Geometry check sheet. Reference: the model listing, model coordinates, mm. Face numbers are marked on the shaded views. A direction names the side the tool comes from. Coordinates: 2 decimals unless noted, no trailing zeros. Loops run counter-clockwise (first coordinate to the right, second up) from the corner with the lowest first, then second, coordinate; pieces in that order, holes last. Notation, with made-up numbers: (68, 33.25) - (87, 33.25) arc R19 cw to (87, 56.25) - close; hole circle Ø9 at (25, -24.5). An arc over 180 degrees is marked (long way). Write each question's results on one line, items separated by ' | '. Start each with the question number.
(1) Sectioned sample at B-B (x = -40). Enter the section's corners in (y, z), plus the area to 3 significant figures.
(2) Access from +Z, -Z, +X, -X, +Y, -Y to the whole of each face (thin tool, end or side, straight path). Record for the marked faces 1, 2 and 3.
(3) Mould release check, pull along X, two halves, no side actions. Record for the marked faces 4, 5 and 6: pulls with the +X half, pulls with the -X half, needs draft (parallel to the pull), parting line crosses it, or undercut.
(4) Go/stop test with flat-tipped pins: pin 1 Ø1 at (x, z) = (-74, 23) entering from -Y; pin 2 Ø13.5 at (y, z) = (-4, 31.5) entering from -X; pin 3 Ø10 at (x, z) = (-61.5, 13.5) entering from -Y. Record where each tip stops, or that it passes through.
(5) Sectioned sample at A-A (y = -24). Enter the section's corners in (x, z), plus the area to 3 significant figures.
(6) Material ranges on probe 1 along Y at (x, z) = (-90, 5.5); probe 2 along X at (y, z) = (-3, 16); probe 3 along X at (y, z) = (-11, 6), recorded low to high.
(7) Sectioned sample at C-C (z = 33). Enter the section's corners in (x, y), plus the area to 3 significant figures.
from build123d import *

# Parameters (mm, degrees)
F1_DEPTH = 40
F2_DEPTH = 10
F3_R     = 3
F4_SIZE  = 0.4
F5_SIZE  = 1


with BuildPart() as f1:
    # F0 (on Top) → F1 (new body)
    with BuildSketch(Plane.XY):
        with BuildLine():
            Line((-32.408465, 29.689309), (-97.408465, 29.689309))
            ThreePointArc((-97.408465, 29.689309), (-100.943999, 28.224843), (-102.408465, 24.689309))
            Line((-102.408465, 24.689309), (-102.408465, -35.310691))
            ThreePointArc((-102.408465, -35.310691), (-100.943999, -38.846224), (-97.408465, -40.310691))
            Line((-97.408465, -40.310691), (-32.408465, -40.310691))
            ThreePointArc((-32.408465, -40.310691), (-28.872931, -38.846224), (-27.408465, -35.310691))
            Line((-27.408465, -35.310691), (-27.408465, 24.689309))
            ThreePointArc((-27.408465, 24.689309), (-28.872931, 28.224843), (-32.408465, 29.689309))
        make_face()
        with BuildLine():
            Line((-101.408465, -34.310691), (-101.408465, 23.689309))
            ThreePointArc((-101.408465, 23.689309), (-99.943999, 27.224843), (-96.408465, 28.689309))
            Line((-96.408465, 28.689309), (-33.408465, 28.689309))
            ThreePointArc((-33.408465, 28.689309), (-29.872931, 27.224843), (-28.408465, 23.689309))
            Line((-28.408465, 23.689309), (-28.408465, -34.310691))
            ThreePointArc((-28.408465, -34.310691), (-29.872931, -37.846224), (-33.408465, -39.310691))
            Line((-33.408465, -39.310691), (-96.408465, -39.310691))
            ThreePointArc((-96.408465, -39.310691), (-99.943999, -37.846224), (-101.408465, -34.310691))
        make_face(mode=Mode.SUBTRACT)
    extrude(amount=F1_DEPTH)

    # F0 (on Top) → F2 (join)
    with BuildSketch(Plane.XY):
        with BuildLine():
            Line((-24.408465, 37.689309), (-105.408465, 37.689309))
            ThreePointArc((-105.408465, 37.689309), (-108.943999, 36.224843), (-110.408465, 32.689309))
            Line((-110.408465, 32.689309), (-110.408465, -43.310691))
            ThreePointArc((-110.408465, -43.310691), (-108.943999, -46.846224), (-105.408465, -48.310691))
            Line((-105.408465, -48.310691), (-24.408465, -48.310691))
            ThreePointArc((-24.408465, -48.310691), (-20.872931, -46.846224), (-19.408465, -43.310691))
            Line((-19.408465, -43.310691), (-19.408465, 32.689309))
            ThreePointArc((-19.408465, 32.689309), (-20.872931, 36.224843), (-24.408465, 37.689309))
        make_face()
        with BuildLine():
            Line((-105.408465, -38.310691), (-105.408465, 27.689309))
            ThreePointArc((-105.408465, 27.689309), (-103.943999, 31.224843), (-100.408465, 32.689309))
            Line((-100.408465, 32.689309), (-29.408465, 32.689309))
            ThreePointArc((-29.408465, 32.689309), (-25.872931, 31.224843), (-24.408465, 27.689309))
            Line((-24.408465, 27.689309), (-24.408465, -38.310691))
            ThreePointArc((-24.408465, -38.310691), (-25.872931, -41.846224), (-29.408465, -43.310691))
            Line((-29.408465, -43.310691), (-100.408465, -43.310691))
            ThreePointArc((-100.408465, -43.310691), (-103.943999, -41.846224), (-105.408465, -38.310691))
        make_face(mode=Mode.SUBTRACT)
        with BuildLine():
            ThreePointArc((-100.408465, 32.689309), (-103.943999, 31.224843), (-105.408465, 27.689309))
            Line((-105.408465, 27.689309), (-105.408465, -38.310691))
            ThreePointArc((-105.408465, -38.310691), (-103.943999, -41.846224), (-100.408465, -43.310691))
            Line((-100.408465, -43.310691), (-29.408465, -43.310691))
            ThreePointArc((-29.408465, -43.310691), (-25.872931, -41.846224), (-24.408465, -38.310691))
            Line((-24.408465, -38.310691), (-24.408465, 27.689309))
            ThreePointArc((-24.408465, 27.689309), (-25.872931, 31.224843), (-29.408465, 32.689309))
            Line((-29.408465, 32.689309), (-100.408465, 32.689309))
        make_face()
        with BuildLine():
            ThreePointArc((-102.408465, 24.689309), (-100.943999, 28.224843), (-97.408465, 29.689309))
            Line((-97.408465, 29.689309), (-32.408465, 29.689309))
            ThreePointArc((-32.408465, 29.689309), (-28.872931, 28.224843), (-27.408465, 24.689309))
            Line((-27.408465, 24.689309), (-27.408465, -35.310691))
            ThreePointArc((-27.408465, -35.310691), (-28.872931, -38.846224), (-32.408465, -40.310691))
            Line((-32.408465, -40.310691), (-97.408465, -40.310691))
            ThreePointArc((-97.408465, -40.310691), (-100.943999, -38.846224), (-102.408465, -35.310691))
            Line((-102.408465, -35.310691), (-102.408465, 24.689309))
        make_face(mode=Mode.SUBTRACT)
    extrude(amount=F2_DEPTH)

    # F3
    f3_edges = [f1.edges().sort_by_distance(p)[0] for p in [
        (-64.908465, -40.310691, 10),
        (-64.908465, -48.310691, 10),
        (-64.908465, -48.310691, 0),
    ]]
    fillet(f3_edges, radius=F3_R)

    # F4
    f4_edges = [f1.edges().sort_by_distance(p)[0] for p in [
        (-64.908465, -40.310691, 40),
        (-64.908465, -39.310691, 40),
    ]]
    chamfer(f4_edges, length=F4_SIZE)

    # F5
    f5_edges = [f1.edges().sort_by_distance(p)[0] for p in [
        (-101.408465, -5.310691, 0),
    ]]
    chamfer(f5_edges, length=F5_SIZE)


solid = f1.part
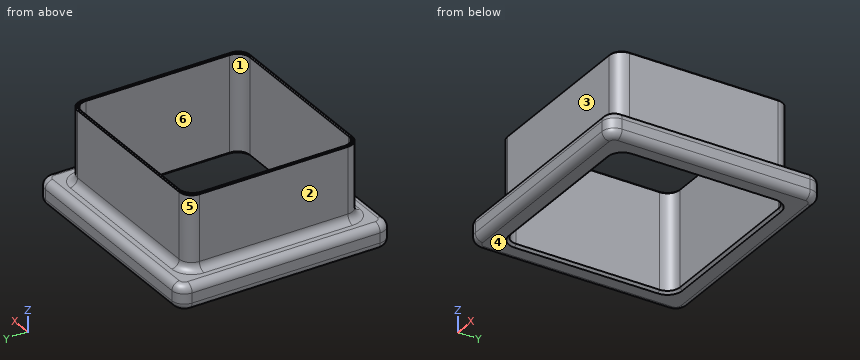
Outcome:
1) outline: (-48.31, 3) arc R3 ccw to (-45.31, 0) - (-40.31, 0) - (-39.31, 1) - (-39.31, 39.6) - (-39.71, 40) - (-39.91, 40) - (-40.31, 39.6) - (-40.31, 13) arc R3 cw to (-43.31, 10) - (-45.31, 10) arc R3 ccw to (-48.31, 7) - close; (28.69, 1) - (29.69, 0) - (34.69, 0) arc R3 ccw to (37.69, 3) - (37.69, 7) arc R3 ccw to (34.69, 10) - (32.69, 10) arc R3 cw to (29.69, 13) - (29.69, 39.6) - (29.29, 40) - (29.09, 40) - (28.69, 39.6) - close | area: 235 mm2
2) face 1: +Z, -Z | face 2: +Z, -X, +Y, -Y | face 3: +Z, +X, -X, -Y
3) face 4: needs draft | face 5: pulls with the -X half | face 6: undercut
4) pin 1: stops at y = -40.31 | pin 2: stops at x = -102.41 | pin 3: stops at y = -47.91
5) outline: (-110.41, 3) arc R3 ccw to (-107.41, 0) - (-102.41, 0) - (-101.41, 1) - (-101.41, 39.6) - (-101.81, 40) - (-102.01, 40) - (-102.41, 39.6) - (-102.41, 13) arc R3 cw to (-105.41, 10) - (-107.41, 10) arc R3 ccw to (-110.41, 7) - close; (-28.41, 1) - (-27.41, 0) - (-22.41, 0) arc R3 ccw to (-19.41, 3) - (-19.41, 7) arc R3 ccw to (-22.41, 10) - (-24.41, 10) arc R3 cw to (-27.41, 13) - (-27.41, 39.6) - (-27.81, 40) - (-28.01, 40) - (-28.41, 39.6) - close | area: 235 mm2
6) probe 1: y = -48.31 to -39.31, 28.69 to 37.69 | probe 2: x = -102.41 to -101.41, -28.41 to -27.41 | probe 3: x = -110.41 to -101.41, -28.41 to -19.41
7) outline: (-102.41, -35.31) arc R5 ccw to (-97.41, -40.31) - (-32.41, -40.31) arc R5 ccw to (-27.41, -35.31) - (-27.41, 24.69) arc R5 ccw to (-32.41, 29.69) - (-97.41, 29.69) arc R5 ccw to (-102.41, 24.69) - close; hole (-101.41, -34.31) arc R5 ccw to (-96.41, -39.31) - (-33.41, -39.31) arc R5 ccw to (-28.41, -34.31) - (-28.41, 23.69) arc R5 ccw to (-33.41, 28.69) - (-96.41, 28.69) arc R5 ccw to (-101.41, 23.69) - close | area: 286 mm2
